Model file for the job. Use its own axes, mm. A direction names the side the tool comes from. Round coordinates to 2 decimals unless told otherwise and drop trailing zeros. Order: outer loops, then holes, each group sorted by start corner. A loop starts at its lowest first (then second) coordinate and runs counter-clockwise, first axis right, second up. Notation, with made-up numbers: (-36, 7.5) -> (-11, 7.5) arc R7 ccw to (-11, 12.5) -> close; hole circle Ø7 at (60, 0.5). An arc over 180 degrees is marked (long way). Answer as CSV lines item,"result".
```python
from build123d import *

# Parameters (mm, degrees)
F0_W     = 140
F0_H     = 50
F1_DEPTH = 5
F2_W     = 12.5
F2_H     = 12.5
F3_DEPTH = 25
F4_R     = 12.5
F5_DEPTH = 25


with BuildPart() as f1:
    # F0 (on Top) → F1 (new body)
    with BuildSketch(Plane.XY):
        with Locations((2.230102, -4.090368)):
            Rectangle(F0_W, F0_H)
    extrude(amount=F1_DEPTH)

    # F2 (on face) → F3 (cut)
    with BuildSketch(Plane.XY.offset(5)):
        with Locations((-56.519898, 10.497632)):
            Rectangle(F2_W, F2_H)
        with Locations((60.980102, 10.497632)):
            Rectangle(F2_W, F2_H)
    extrude(amount=-F3_DEPTH, mode=Mode.SUBTRACT)

    # F4 (on face) → F5 (cut)
    with BuildSketch(Plane.XY.offset(5)):
        with Locations((2.230102, -11.590368)):
            Circle(F4_R)
    extrude(amount=-F5_DEPTH, mode=Mode.SUBTRACT)


solid = f1.part
```
Q1. Tool access for faces 4 (the flat face through (61, 4.248, 3)), 5 (the flat face through (1, -29.09, 2)): list every direction of +Z, -Z, +X, -X, +Y, -Y with a clear straight run to the whole face (end or side of a thin tool).
Checks:
face 4,"+Z, -Z"
face 5,"+Z, -Z, +X, -X, -Y"
Q2. Saw through at C-C (z = 3.05). Write the cut outline in (x, y), plus the area to 3 significant figures.
Checks:
outline,"(-67.77, -29.09) -> (72.23, -29.09) -> (72.23, 20.91) -> (-67.77, 20.91) -> close; hole (-62.77, 4.25) -> (-50.27, 4.25) -> (-50.27, 16.75) -> (-62.77, 16.75) -> close; hole circle Ø25 at (2.23, -11.59); hole (54.73, 4.25) -> (67.23, 4.25) -> (67.23, 16.75) -> (54.73, 16.75) -> close"
area,"6,200 mm²"
Q3. Wall check: L1, parallel to X at y = 11.5, z = 3.4; L2, parallel to Y at x = -54, z = 1.65; L3, parallel to X at y = -17, z = 3.9. Give the ranges that are in metal, low to high. Write a range as [from, to].
Checks:
L1,"[-67.77, -62.77], [-50.27, 54.73], [67.23, 72.23]"
L2,"[-29.09, 4.25], [16.75, 20.91]"
L3,"[-67.77, -9.04], [13.5, 72.23]"
Q4. Saw through at D-D (y = -4.5). Write the cut outline in (x, z), plus the area to 3 significant figures.
Checks:
outline,"(-67.77, 0) -> (-8.06, 0) -> (-8.06, 5) -> (-67.77, 5) -> close; (12.52, 0) -> (72.23, 0) -> (72.23, 5) -> (12.52, 5) -> close"
area,"597 mm²"
Q5. Saw through at A-A (y = 7). Write the cut outline in (x, z), plus the area to 3 significant figures.
Checks:
outline,"(-67.77, 0) -> (-62.77, 0) -> (-62.77, 5) -> (-67.77, 5) -> close; (-50.27, 0) -> (54.73, 0) -> (54.73, 5) -> (-50.27, 5) -> close; (67.23, 0) -> (72.23, 0) -> (72.23, 5) -> (67.23, 5) -> close"
area,"575 mm²"
Q6. Saw through at B-B (x = -4.5). Write the cut outline in (y, z), plus the area to 3 significant figures.
Checks:
outline,"(-29.09, 0) -> (-22.12, 0) -> (-22.12, 5) -> (-29.09, 5) -> close; (-1.06, 0) -> (20.91, 0) -> (20.91, 5) -> (-1.06, 5) -> close"
area,"145 mm²"
Q7. Flat gauge pin, fed straight in: pin 1 (1 mm diameter, centred on x = -2, y = 0, fed in from -Z). Where does the tip first touch, or does it go through?
Checks:
pin 1,"z = 0"
Q8. Mould opens along Y. For faces 1 (the flat face through (1, 2, 0)), 2 (the flat face through (-57, 4.248, 3)), 3 (the flat face through (1, 20.91, 2)) say: +Y half, -Y half, draft (parallel to the pull), parting line (faces both ways), or undercut.
Checks:
face 1,"draft"
face 2,"undercut"
face 3,"+Y half"
